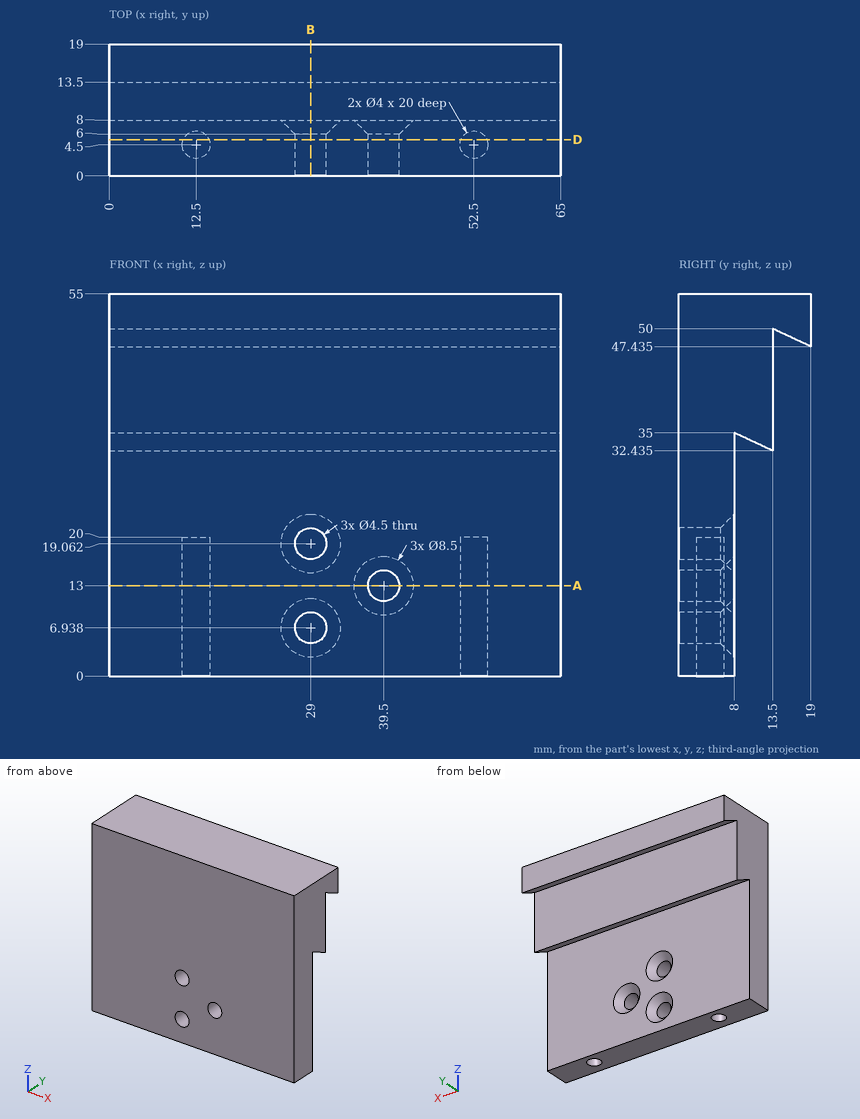
Design review of the part shown in the three views and the two pictorial views. Dimensions are in mm from the part's minimum x, y and z. Give positions to 0.01 mm unless a question says otherwise; leave off trailing zeros. Loops run counter-clockwise (first coordinate to the right, second up) from the corner with the lowest first, then second, coordinate; pieces in that order, holes last. Notation, with made-up numbers: (-11.5, 39.25) -> (47.5, 39.25) arc R15 cw to (47.5, 46.25) -> close; hole circle Ø10 at (67, -25). An arc over 180 degrees is marked (long way). Answer as a JSON object with one key per item and string values. Group by question number.
Q1. Take a section at D-D (y = 5.25). Write out the cut boundary in (x, z), plus the area to 3 significant figures.
Q2. Wall thickness on line 1 along Y through (x, z) = (52.5, 11.5); line 2 along X through (y, z) = (4.05, 13); line 3 along Z through (x, y) = (30, 2.5): over which ranges is each line inside the solid? List them lowest first.
Q3. Take a section at B-B (x = 29). Write out the cut boundary in (y, z) (1 decimal), plus the area to 3 significant figures.
Q4. Insertion check: pin 1 (3 mm diameter, centred on x = 12.5, y = 4.5, fed in from -Z); pin 2 (2 mm diameter, centred on x = 50, z = 26, fed in from +Y); pin 3 (5.5 mm diameter, centred on x = 41.5, z = 39, fed in from +Y). Each pin has a flat end and moves straight along its axis. Give the tip position at first contact, or say it passes through.
Q5. Take a section at A-A (z = 13). Write out the cut boundary in (x, y).
Answer below:
{
 "1": {"outline": "(0, 0) -> (10.65, 0) -> (10.65, 20) -> (14.35, 20) -> (14.35, 0) -> (50.65, 0) -> (50.65, 20) -> (54.35, 20) -> (54.35, 0) -> (65, 0) -> (65, 55) -> (0, 55) -> close; hole circle Ø4.5 at (29, 6.94); hole circle Ø4.5 at (29, 19.06); hole circle Ø4.5 at (39.5, 13)", "area": "3,380 mm2"},
 "2": {"line 1": "y = 0 to 2.5, 6.5 to 8", "line 2": "x = 0 to 10.55, 14.45 to 37.25, 41.75 to 50.55, 54.45 to 65", "line 3": "z = 0 to 4.92, 8.95 to 17.05, 21.08 to 55"},
 "3": {"outline": "(0, 0) -> (8, 0) -> (8, 2.7) -> (6, 4.7) -> (0, 4.7) -> close; (0, 9.2) -> (6, 9.2) -> (8, 11.2) -> (8, 14.8) -> (6, 16.8) -> (0, 16.8) -> close; (0, 21.3) -> (6, 21.3) -> (8, 23.3) -> (8, 35) -> (13.5, 32.4) -> (13.5, 50) -> (19, 47.4) -> (19, 55) -> (0, 55) -> close", "area": "512 mm2"},
 "4": {"pin 1": "stops at z = 20", "pin 2": "stops at y = 8", "pin 3": "stops at y = 13.5"},
 "5": {"outline": "(0, 0) -> (37.25, 0) -> (37.25, 6) -> (35.25, 8) -> (0, 8) -> close; (41.75, 0) -> (65, 0) -> (65, 8) -> (43.75, 8) -> (41.75, 6) -> close; hole circle Ø4 at (12.5, 4.5); hole circle Ø4 at (52.5, 4.5)"}
}
